```python
from build123d import *

# Parameters (mm, degrees)
SKETCH1_W                                           = 140
SKETCH1_H                                           = 65
BOSS_EXTRUDE1_DEPTH                                 = 30
SKETCH2_R                                           = 7.5
SKETCH2_R_2                                         = 3.25
CUT_EXTRUDE2_DEPTH                                  = 27
SKETCH4_R                                           = 7.5
CUT_EXTRUDE3_DEPTH                                  = 82.76337811
SKETCH5_R                                           = 5
CUT_EXTRUDE4_DEPTH                                  = 83.802475808
SKETCH6_W                                           = 3
SKETCH6_H                                           = 37
CUT_EXTRUDE5_DEPTH                                  = 83.802475808
CBORE_FOR_M5_HEX_SOCKET_HEAD_CAP_SCREW1_D           = 5.5
CBORE_FOR_M5_HEX_SOCKET_HEAD_CAP_SCREW1_DEPTH       = 8.5
CBORE_FOR_M5_HEX_SOCKET_HEAD_CAP_SCREW1_CBORE_D     = 10
CBORE_FOR_M5_HEX_SOCKET_HEAD_CAP_SCREW1_CBORE_DEPTH = 5.4
TAP_DRILL_FOR_M5_TAP1_AT_2_COUNT                    = 2
TAP_DRILL_FOR_M5_TAP1_AT_2_PITCH                    = 18
CBORE_FOR_M6_HEX_SOCKET_HEAD_CAP_SCREW3_D           = 6.6
CBORE_FOR_M6_HEX_SOCKET_HEAD_CAP_SCREW3_CBORE_D     = 11
CBORE_FOR_M6_HEX_SOCKET_HEAD_CAP_SCREW3_CBORE_DEPTH = 61.4
CIRPATTERN1_COUNT                                   = 4
SKETCH29_W                                          = 35
SKETCH29_H                                          = 2
CUT_EXTRUDE6_DEPTH                                  = 83.802475808
CHAMFER2_SIZE                                       = 10
SKETCH2_2_R                                         = 7.5
SKETCH2_2_R_2                                       = 3.25
CUT_EXTRUDE7_DEPTH                                  = 83.802475808


with BuildPart() as part:
    # Sketch1 → Boss-Extrude1 (new body)
    with BuildSketch(Plane.XY):
        Rectangle(SKETCH1_W, SKETCH1_H)
    extrude(amount=BOSS_EXTRUDE1_DEPTH)

    # Sketch2 → Cut-Extrude2 (cut)
    with BuildSketch(Plane(origin=(0, 0, 30), x_dir=(-1, 0, 0), z_dir=(0, 0, -1))):
        with Locations((0, -2.5)):
            Circle(SKETCH2_R)
        with Locations((24, -2.5)):
            Circle(SKETCH2_R_2)
        with Locations(Location((-24, -2.5, 0), (0, 0, 180))):
            Circle(SKETCH2_R_2)
    extrude(amount=CUT_EXTRUDE2_DEPTH, mode=Mode.SUBTRACT)

    # Sketch4 → Cut-Extrude3 (cut, through all)
    with BuildSketch(Plane.XY.offset(3)):
        with Locations((0, -2.5)):
            Circle(SKETCH4_R)
    extrude(amount=-CUT_EXTRUDE3_DEPTH, mode=Mode.SUBTRACT)

    # Sketch5 → Cut-Extrude4 (cut, through all)
    with BuildSketch(Plane(origin=(0, 0, 0), x_dir=(-1, 0, 0), z_dir=(0, 0, -1))):
        with Locations((-60, 7.5)):
            Circle(SKETCH5_R)
        with Locations((60, 7.5)):
            Circle(SKETCH5_R)
    extrude(amount=-CUT_EXTRUDE4_DEPTH, mode=Mode.SUBTRACT)

    # Sketch6 → Cut-Extrude5 (cut, through all)
    with BuildSketch(Plane(origin=(0, 0, 0), x_dir=(-1, 0, 0), z_dir=(0, 0, -1))):
        with Locations((-60, 14)):
            Rectangle(SKETCH6_W, SKETCH6_H)
        with Locations((60, 14)):
            Rectangle(SKETCH6_W, SKETCH6_H)
    extrude(amount=-CUT_EXTRUDE5_DEPTH, mode=Mode.SUBTRACT)

    # CBORE for M5 Hex Socket Head Cap Screw1
    with Locations(Plane(origin=(70, 0, 0), x_dir=(0, 0, -1), z_dir=(1, 0, 0))):
        with Locations((-6, 22.5), (-24, 22.5)):
            cbore_for_m5_hex_socket_head_cap_screw1 = CounterBoreHole(CBORE_FOR_M5_HEX_SOCKET_HEAD_CAP_SCREW1_D / 2, CBORE_FOR_M5_HEX_SOCKET_HEAD_CAP_SCREW1_CBORE_D / 2, CBORE_FOR_M5_HEX_SOCKET_HEAD_CAP_SCREW1_CBORE_DEPTH, depth=CBORE_FOR_M5_HEX_SOCKET_HEAD_CAP_SCREW1_DEPTH)

    # Sketch12 → Tap Drill for M5 Tap1 (revolve, cut)
    with BuildSketch(Plane(origin=(58.5, 22.5, 6), x_dir=(0, 0, -1), z_dir=(0, 1, 0))):
        Polygon((0, 0), (0, 13.2618073), (2.1, 12), (2.1, 0), align=None)
    tap_drill_for_m5_tap1 = revolve(axis=Axis((64.85, 22.5, 6), (-1, 0, 0)), mode=Mode.SUBTRACT)

    # Tap Drill for M5 Tap1 at 2: Tap Drill for M5 Tap1 ×2
    with Locations(*[(0, 0, i * TAP_DRILL_FOR_M5_TAP1_AT_2_PITCH) for i in range(1, TAP_DRILL_FOR_M5_TAP1_AT_2_COUNT)]):
        add(tap_drill_for_m5_tap1, mode=Mode.SUBTRACT)

    # Sketch15 → Tap Drill for M6 Tap1 (revolve, cut)
    with BuildSketch(Plane(origin=(70, -17.5, 15), x_dir=(0, 0, -1), z_dir=(0, 1, 0))):
        Polygon((0, 0), (0, 16.502151548), (2.5, 15), (2.5, 0), align=None)
    tap_drill_for_m6_tap1 = revolve(axis=Axis((76.35, -17.5, 15), (-1, 0, 0)), mode=Mode.SUBTRACT)

    # Mirror1: CBORE for M5 Hex Socket Head Cap Screw1, Tap Drill for M5 Tap1, Tap Drill for M6 Tap1 across plane
    add(cbore_for_m5_hex_socket_head_cap_screw1.mirror(Plane(origin=(0, 0, 0), x_dir=(0, 0, 1), z_dir=(1, 0, 0))), mode=Mode.SUBTRACT)
    add(tap_drill_for_m5_tap1.mirror(Plane(origin=(0, 0, 0), x_dir=(0, 0, 1), z_dir=(1, 0, 0))), mode=Mode.SUBTRACT)
    add(tap_drill_for_m6_tap1.mirror(Plane(origin=(0, 0, 0), x_dir=(0, 0, 1), z_dir=(1, 0, 0))), mode=Mode.SUBTRACT)

    # Mirror1 copy 1 sketch → Mirror1 copy 1 (revolve, cut)
    with BuildSketch(Plane(origin=(-58.5, 22.5, 24), x_dir=(0, 0, -1), z_dir=(0, 1, 0))):
        Polygon((0, 0), (0, -13.2618073), (2.1, -12), (2.1, 0), align=None)
    revolve(axis=Axis((-64.85, 22.5, 24), (-1, 0, 0)), mode=Mode.SUBTRACT)

    # CBORE for M6 Hex Socket Head Cap Screw3 (through all)
    with Locations(Plane(origin=(0, 32.5, 0), x_dir=(1, 0, 0), z_dir=(0, 1, 0))):
        with Locations((40, -15), (-40, -15)):
            CounterBoreHole(CBORE_FOR_M6_HEX_SOCKET_HEAD_CAP_SCREW3_D / 2, CBORE_FOR_M6_HEX_SOCKET_HEAD_CAP_SCREW3_CBORE_D / 2, CBORE_FOR_M6_HEX_SOCKET_HEAD_CAP_SCREW3_CBORE_DEPTH)

    # Sketch28 → Tap Drill for M4 Tap1 (revolve, cut)
    with BuildSketch(Plane(origin=(0, 22.5, 30), x_dir=(0, -1, 0), z_dir=(1, 0, 0))):
        Polygon((0, 0), (0, 8.991420021), (1.65, 8), (1.65, 0), align=None)
    tap_drill_for_m4_tap1 = revolve(axis=Axis((0, 22.5, 36.35), (0, 0, -1)), mode=Mode.SUBTRACT)

    # CirPattern1: Tap Drill for M4 Tap1 ×4 about axis, 2 skipped
    cirpattern1_axis = Axis((0, -2.5, 3), (0, 0, 1))
    add([tap_drill_for_m4_tap1.rotate(cirpattern1_axis, i * 360 / CIRPATTERN1_COUNT) for i in range(1, CIRPATTERN1_COUNT) if i not in (1, 3)], mode=Mode.SUBTRACT)

    # Sketch29 → Cut-Extrude6 (cut, through all)
    with BuildSketch(Plane.XY.offset(30)):
        with Locations((0, -31.5)):
            Rectangle(SKETCH29_W, SKETCH29_H)
    extrude(amount=-CUT_EXTRUDE6_DEPTH, mode=Mode.SUBTRACT)

    # Chamfer2
    # the kernel refuses this chamfer: 10 mm, written as the material it adds along each edge
    with BuildSketch(Plane(origin=(-17.5, -30.5, 30), x_dir=(-0.02749587661058977, -0.9996219169112965, 0), z_dir=(0, 0, -1))) as chamfer2_piece_1_section:
        Polygon((CHAMFER2_SIZE * 0.999621916911, -CHAMFER2_SIZE * 0.0274958766106), (-CHAMFER2_SIZE * 0.0274958766106, -CHAMFER2_SIZE * 0.999621916911), (0, 0), align=None)
    chamfer2_piece_1 = extrude(amount=30, mode=Mode.PRIVATE)
    chamfer2_piece_1 = split(chamfer2_piece_1, bisect_by=Plane(origin=(-12.880949734, -32.5, 15), z_dir=(0, 1, 0)), keep=Keep.TOP, mode=Mode.PRIVATE)
    add(chamfer2_piece_1)
    with BuildSketch(Plane(origin=(17.5, -30.5, 30), x_dir=(-0.9996219169112968, 0.027495876610586317, 0), z_dir=(0, 0, -1))) as chamfer2_piece_2_section:
        Polygon((CHAMFER2_SIZE * 0.999621916911, -CHAMFER2_SIZE * 0.0274958766106), (-CHAMFER2_SIZE * 0.0274958766106, -CHAMFER2_SIZE * 0.999621916911), (0, 0), align=None)
    chamfer2_piece_2 = extrude(amount=30, mode=Mode.PRIVATE)
    chamfer2_piece_2 = split(chamfer2_piece_2, bisect_by=Plane(origin=(12.880949734, -32.5, 15), z_dir=(0, 1, 0)), keep=Keep.TOP, mode=Mode.PRIVATE)
    add(chamfer2_piece_2)

    # Sketch2<2> → Cut-Extrude7 (cut, through all)
    with BuildSketch(Plane(origin=(0, 0, 30), x_dir=(-1, 0, 0), z_dir=(0, 0, -1))):
        with Locations(Location((0, -2.5, 0), (0, 0, 180))):
            Circle(SKETCH2_2_R)
        with Locations((24, -2.5)):
            Circle(SKETCH2_2_R_2)
        with Locations(Location((-24, -2.5, 0), (0, 0, 180))):
            Circle(SKETCH2_2_R_2)
    extrude(amount=CUT_EXTRUDE7_DEPTH, mode=Mode.SUBTRACT)


solid = part.part
```
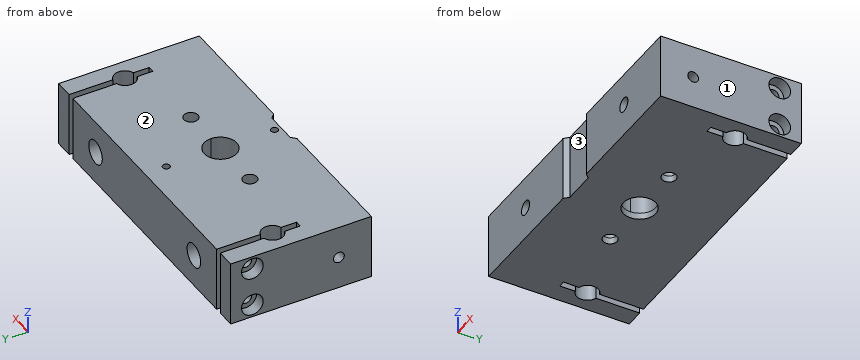
The model under review builds one solid part; all positions refer to its coordinate system, in mm. Face numbers are marked on the shaded views. Coordinates: 2 decimals unless noted, no trailing zeros. Write each loop counter-clockwise with the first axis right and the second up, starting at its lowest first coordinate (ties: lowest second). Pieces come first, ordered by that corner, then holes.
1) We need section C-C on x = -24. State the section outline as (y, z) points, then the cut area to 4 significant figures.
2) The part is to be moulded in two halves that separate along X. For the marked faces 1, 2 and 3, say which applies: pulls with the +X half, pulls with the -X half, needs draft (parallel to the pull), parting line crosses it, or undercut.
3) We need section B-B on y = -24.5. State the section outline as (x, z) points, then the cut area to 3 significant figures.
4) Clearance check with flat-ended pins moving along their axes: pin 1 Ø4 at (y, z) = (22.5, 6) entering from +X; pin 2 Ø4 at (y, z) = (22.5, 6) entering from -X; pin 3 Ø6 at (y, z) = (22.5, 24) entering from +X; pin 4 Ø4 at (x, y) = (-24, -2.5) entering from -Z. State where each tip first meets the part, or that it passes through.
5) We need section A-A on x = 40. State the section outline as (y, z) points.
6) We need section D-D on x = 6. State the section outline as (y, z) points.
7) To check wall thickness, follow probe 1 along Z at (x, y) = (-66.45, 22.5); probe 2 along Z at (x, y) = (-65.25, -17.5); probe 3 along X at (y, z) = (14, 9). State the ranges of each line that lie inside material, in increasing order.
Answer list:
1. outline: (-32.5, 0) - (-5.75, 0) - (-5.75, 30) - (-32.5, 30) - close; (0.75, 0) - (32.5, 0) - (32.5, 30) - (0.75, 30) - close
1. area: 1,755 mm2
2. face 1: pulls with the +X half
2. face 2: needs draft
2. face 3: undercut
3. outline: (-70, 0) - (70, 0) - (70, 30) - (-70, 30) - close; hole circle Ø11 at (-40, 15); hole circle Ø11 at (40, 15)
3. area: 4,010 mm2
4. pin 1: stops at x = 46.44
4. pin 2: stops at x = -46.44
4. pin 3: stops at x = 64.6
4. pin 4: passes through
5. outline: (-32.5, 0) - (32.5, 0) - (32.5, 9.5) - (-28.9, 9.5) - (-28.9, 11.7) - (-32.5, 11.7) - close; (-32.5, 18.3) - (-28.9, 18.3) - (-28.9, 20.5) - (32.5, 20.5) - (32.5, 30) - (-32.5, 30) - close
6. outline: (-30.5, 0) - (-7, 0) - (-7, 30) - (-30.5, 30) - close; (2, 0) - (32.5, 0) - (32.5, 30) - (2, 30) - close
7. probe 1: z = 0 to 1, 11 to 19, 29 to 30
7. probe 2: z = 0 to 12.5, 17.5 to 30
7. probe 3: x = -70 to -61.5, -58.5 to 58.5, 61.5 to 70
